```python
from build123d import *

# Parameters (mm, degrees)
SKETCH_1_W          = 88
SKETCH_1_H          = 100
EXTRUDE_1_DEPTH     = 4
SKETCH_2_R          = 2
CUT_EXTRUDE_1_DEPTH = 67.72330927
SKETCH_3_R          = 2.5
CUT_EXTRUDE_2_DEPTH = 67.72330927


with BuildPart() as part:
    # 草图1 → 凸台-拉伸1 (new body)
    with BuildSketch(Plane.XY):
        Rectangle(SKETCH_1_W, SKETCH_1_H)
    extrude(amount=EXTRUDE_1_DEPTH)

    # 草图2 → 切除-拉伸1 (cut, through all)
    with BuildSketch(Plane.XY.offset(4)):
        with Locations((-36.5, 42.5)):
            Circle(SKETCH_2_R)
        with Locations((36.5, 42.5)):
            Circle(SKETCH_2_R)
        with Locations((36.5, -42.5)):
            Circle(SKETCH_2_R)
        with Locations((-36.5, -42.5)):
            Circle(SKETCH_2_R)
    extrude(amount=-CUT_EXTRUDE_1_DEPTH, mode=Mode.SUBTRACT)

    # 草图3 → 切除-拉伸2 (cut, through all)
    with BuildSketch(Plane.XY.offset(4)):
        with Locations((-15, 25)):
            Circle(SKETCH_3_R)
        with Locations((15, 25)):
            Circle(SKETCH_3_R)
        with Locations((15, -5)):
            Circle(SKETCH_3_R)
        with Locations((-15, -5)):
            Circle(SKETCH_3_R)
    extrude(amount=-CUT_EXTRUDE_2_DEPTH, mode=Mode.SUBTRACT)


solid = part.part
```
Work out the finished part from the listing and answer in its coordinate system (mm). Round coordinates to 2 decimals unless told otherwise and drop trailing zeros. Write each loop counter-clockwise with the first axis right and the second up, starting at its lowest first coordinate (ties: lowest second). Pieces come first, ordered by that corner, then holes. Notation, with made-up numbers: (-9, -5.5) -> (20, -5.5) arc R31 ccw to (20, 26.5) -> close; hole circle Ø4 at (56, -15). An arc over 180 degrees is marked (long way). Write each question's results on one line, items separated by ' | '.
1) The part is cut by section A-A (y = 25). Write down the section's boundary in (x, z).
Findings:
outline: (-44, 0) -> (-17.5, 0) -> (-17.5, 4) -> (-44, 4) -> close; (-12.5, 0) -> (12.5, 0) -> (12.5, 4) -> (-12.5, 4) -> close; (17.5, 0) -> (44, 0) -> (44, 4) -> (17.5, 4) -> close
2) Consider line 1 along Y through (x, z) = (36.5, 2.2); line 2 along Y through (x, z) = (15, 2.8); line 3 along X through (y, z) = (-6.5, 1.9). Determine where each line is inside the solid, lowest interval first. Write a range as [from, to].
Findings:
line 1: y = [-50, -44.5], [-40.5, 40.5], [44.5, 50] | line 2: y = [-50, -7.5], [-2.5, 22.5], [27.5, 50] | line 3: x = [-44, -17], [-13, 13], [17, 44]
3) The part is cut by section B-B (x = 15). Write down the section's boundary in (y, z), and give its area (3 significant figures).
Findings:
outline: (-50, 0) -> (-7.5, 0) -> (-7.5, 4) -> (-50, 4) -> close; (-2.5, 0) -> (22.5, 0) -> (22.5, 4) -> (-2.5, 4) -> close; (27.5, 0) -> (50, 0) -> (50, 4) -> (27.5, 4) -> close | area: 360 mm²
4) Flat-ended cylindrical pins translate along their axes: pin 1 (2.5 mm diameter, centred on x = -36.5, y = 42.5, fed in from -Z); pin 2 (5 mm diameter, centred on x = -36.5, y = -42.5, fed in from +Z). Find the tip coordinate at first contact, or state that the pin passes through.
Findings:
pin 1: passes through | pin 2: stops at z = 4
5) For a pull along X with two mould halves and no side action, classify faces 1 (the flat face through (-1, 1, 0)), 2 (the flat face through (44, -1, 2)), 3 (the cylindrical face through (-36.934, 40.548, 2.028)) as +X half, -X half, draft (parallel to the pull), parting line (faces both ways), or undercut.
Findings:
face 1: draft | face 2: +X half | face 3: undercut
